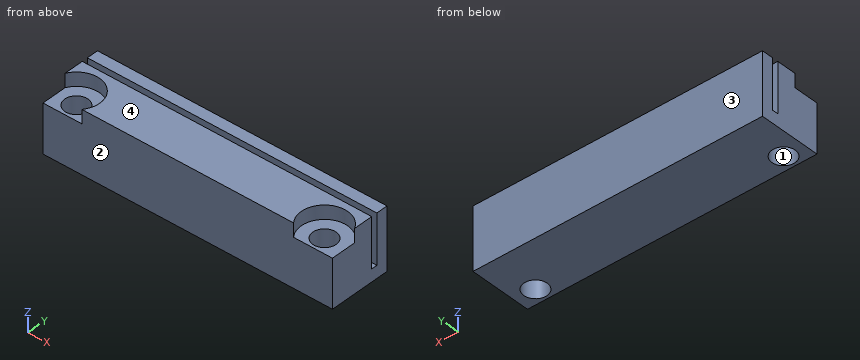
from build123d import *

# Parameters (mm, degrees)
SKETCH1_W                                            = 88.9
SKETCH1_H                                            = 19.05
BOSS_EXTRUDE1_DEPTH                                  = 19.05
CBORE_FOR_1_4_BINDING_HEAD_MACHINE_SCREW_D           = 7.14248
CBORE_FOR_1_4_BINDING_HEAD_MACHINE_SCREW_CBORE_D     = 14.2875
CBORE_FOR_1_4_BINDING_HEAD_MACHINE_SCREW_CBORE_DEPTH = 4.191
SKETCH5_W                                            = 98.267434004
SKETCH5_H                                            = 1.8
CUT_EXTRUDE1_DEPTH                                   = 15.24
SKETCH6_R                                            = 6.169746407
SKETCH6_R_2                                          = 8.762598039
CUT_EXTRUDE2_DEPTH                                   = 15.24


with BuildPart() as part:
    # Sketch1 → Boss-Extrude1 (new body)
    with BuildSketch(Plane.XY):
        Rectangle(SKETCH1_W, SKETCH1_H)
    extrude(amount=BOSS_EXTRUDE1_DEPTH)

    # CBORE for 1/4 Binding Head Machine Screw1 (through all)
    with Locations(Plane.XY.offset(19.05)):
        with Locations((-38.1, -5.08), (38.1, -5.08)):
            CounterBoreHole(CBORE_FOR_1_4_BINDING_HEAD_MACHINE_SCREW_D / 2, CBORE_FOR_1_4_BINDING_HEAD_MACHINE_SCREW_CBORE_D / 2, CBORE_FOR_1_4_BINDING_HEAD_MACHINE_SCREW_CBORE_DEPTH)

    # Sketch5 → Cut-Extrude1 (cut)
    with BuildSketch(Plane.XY.offset(19.05)):
        with Locations((0, 5.08)):
            Rectangle(SKETCH5_W, SKETCH5_H)
    extrude(amount=-CUT_EXTRUDE1_DEPTH, mode=Mode.SUBTRACT)

    # Sketch6 → Cut-Extrude2 (cut)
    with BuildSketch(Plane.XY.offset(14.859)):
        with Locations((-47.154600555, -9.207193904)):
            Circle(SKETCH6_R)
        with Locations((49.650008249, -12.821232633)):
            Circle(SKETCH6_R_2)
    extrude(amount=CUT_EXTRUDE2_DEPTH, mode=Mode.SUBTRACT)


solid = part.part
Input: part model. Units: mm. Frame: model coordinates. Face numbers are marked on the shaded views. Give positions to 0.01 mm unless a question says otherwise; leave off trailing zeros. Write each loop counter-clockwise with the first axis right and the second up, starting at its lowest first coordinate (ties: lowest second). Pieces come first, ordered by that corner, then holes. Notation, with made-up numbers: M 68,56 L 81,56 A25 cw 81,74 Z; hole C -10.75,6.25 d9. An arc over 180 degrees is marked long. Write item = value, one per line. Start each with the question number.
1) First-contact query: pin 1 Ø9.5 at (x, y) = (-35, -6) entering from +Z; pin 2 Ø1.4 at (x, y) = (3, 5) entering from +Z; pin 3 Ø8.5 at (x, y) = (-38.1, -5.08) entering from +Z. Flat tips, straight axial feed; report the tip coordinate or a pass-through.
2) Cut plane D-D on x = -22. Return the cut outline in (y, z) (3 decimals).
3) Cut plane C-C on x = 38.1. Return the cut outline in (y, z) (3 decimals), then the cut area to 3 significant figures.
4) Material intervals for line 1 along Y through (x, z) = (38.1, 10.75) (3 decimals); line 2 along Y through (x, z) = (-30, 12) (3 decimals); line 3 along X through (y, z) = (-6.75, 8), sorted ascending. Write a range as [from, to].
5) Draft query along Y for the marked faces 1, 2, 3 and 4. Return one class per face: +Y half, -Y half, draft (parallel to the pull), parting line (faces both ways), or undercut.
6) Cut plane B-B on y = -5.08. Return the cut outline in (x, z).
7) Cut plane A-A on z = 12.25. Return the cut outline in (x, y) (3 decimals), then the cut area to 3 significant figures.
Solved:
q1.pin_1 = 19.05
q1.pin_2 = 3.81
q1.pin_3 = 14.86
q2.outline = M -9.525,0 L 9.525,0 L 9.525,19.05 L 5.98,19.05 L 5.98,3.81 L 4.18,3.81 L 4.18,19.05 L -9.525,19.05 Z
q3.outline = M -9.525,0 L -8.651,0 L -8.651,14.859 L -9.525,14.859 Z; M -1.509,0 L 9.525,0 L 9.525,19.05 L 5.98,19.05 L 5.98,3.81 L 4.18,3.81 L 4.18,19.05 L 2.064,19.05 L 2.064,14.859 L -1.509,14.859 Z
q3.area = 181 mm2
q4.line_1 = [-9.525, -8.651], [-1.509, 4.18], [5.98, 9.525]
q4.line_2 = [-9.525, 4.18], [5.98, 9.525]
q4.line_3 = [-44.45, -41.26], [-34.94, 34.94], [41.26, 44.45]
q5.face_1 = undercut
q5.face_2 = -Y half
q5.face_3 = +Y half
q5.face_4 = draft
q6.outline = M -44.45,0 L -41.67,0 L -41.67,14.86 L -44.45,14.86 Z; M -34.53,0 L 34.53,0 L 34.53,14.86 L 30.96,14.86 L 30.96,19.05 L -30.96,19.05 L -30.96,14.86 L -34.53,14.86 Z; M 41.67,0 L 44.45,0 L 44.45,14.86 L 41.67,14.86 Z
q7.outline = M -44.45,-9.525 L 44.45,-9.525 L 44.45,4.18 L -44.45,4.18 Z; M -44.45,5.98 L 44.45,5.98 L 44.45,9.525 L -44.45,9.525 Z; hole C -38.1,-5.08 d7.142; hole C 38.1,-5.08 d7.142
q7.area = 1,450 mm2
